CAD build for the part. Positions are in the model's coordinates, mm. A direction names the side the tool comes from. Give positions to 0.01 mm unless a question says otherwise; leave off trailing zeros. Write each loop counter-clockwise with the first axis right and the second up, starting at its lowest first coordinate (ties: lowest second). Pieces come first, ordered by that corner, then holes. Notation, with made-up numbers: (-33.5, 12.5) - (-8.5, 12.5) arc R13 cw to (-8.5, 32.5) - close; hole circle Ø7 at (44, 25.5). An arc over 180 degrees is marked (long way). Answer as a JSON object with one key per item and string values.
from build123d import *

# Parameters (mm, degrees)
SKETCH1_W           = 120
SKETCH1_H           = 40
BOSS_EXTRUDE1_DEPTH = 40
SHELL1_T            = -2
SKETCH2_R           = 18
CUT_EXTRUDE1_DEPTH  = 3
CUT_EXTRUDE2_REACH  = 42
SKETCH3_W           = 30
SKETCH3_H           = 36


with BuildPart() as part:
    # Sketch1 → Boss-Extrude1 (new body)
    with BuildSketch(Plane(origin=(0, 0, 0), x_dir=(1, 0, 0), z_dir=(0, 1, 0))):
        with Locations((-60, 20)):
            Rectangle(SKETCH1_W, SKETCH1_H)
    extrude(amount=BOSS_EXTRUDE1_DEPTH)

    # Shell1
    shell1_openings = [part.faces().sort_by_distance(p)[0] for p in [
        (-120, 20, -20),
    ]]
    offset(amount=SHELL1_T, openings=shell1_openings, kind=Kind.INTERSECTION)

    # Sketch2 → Cut-Extrude1 (cut, through all)
    with BuildSketch(Plane(origin=(0, 2, 0), x_dir=(1, 0, 0), z_dir=(0, 1, 0))):
        with Locations((-20, 20)):
            Circle(SKETCH2_R)
    extrude(amount=-CUT_EXTRUDE1_DEPTH, mode=Mode.SUBTRACT)

    # Sketch3 → Cut-Extrude2 (cut, up to next)
    with BuildSketch(Plane(origin=(0, 40, 0), x_dir=(1, 0, 0), z_dir=(0, 1, 0)), mode=Mode.PRIVATE) as cut_extrude2_sk1:
        with Locations((-101, 20)):
            Rectangle(SKETCH3_W, SKETCH3_H)
    cut_extrude2_tool1 = extrude(cut_extrude2_sk1.sketch, amount=-CUT_EXTRUDE2_REACH, mode=Mode.PRIVATE) & part.part
    add(cut_extrude2_tool1.solids().sort_by_distance((-101, 40, -20))[0], mode=Mode.SUBTRACT)


solid = part.part
Item 1: Cut at A-A (x = -96.5). Give the cut face in (y, z).
Entries:
{"outline": "(0, -40) - (40, -40) - (40, -38) - (2, -38) - (2, -2) - (40, -2) - (40, 0) - (0, 0) - close"}
Item 2: Mould opens along Y. For faces 5 (the flat face through (-6, 2, -6)), 6 (the flat face through (-61, 20, -40)), 7 (the flat face through (-48, 40, -20)) say: +Y half, -Y half, draft (parallel to the pull), parting line (faces both ways), or undercut.
Entries:
{"face 5": "undercut", "face 6": "draft", "face 7": "+Y half"}
Item 3: Cut at C-C (y = 32.5). Give the cut face in (x, z), and give its area (3 significant figures).
Entries:
{"outline": "(-120, -40) - (0, -40) - (0, 0) - (-120, 0) - (-120, -2) - (-2, -2) - (-2, -38) - (-120, -38) - close", "area": "552 mm2"}
Item 4: Cut at D-D (x = -58). Give the cut face in (y, z), and give its area (3 significant figures).
Entries:
{"outline": "(0, -40) - (40, -40) - (40, 0) - (0, 0) - close; hole (2, -38) - (38, -38) - (38, -2) - (2, -2) - close", "area": "304 mm2"}
Item 5: Probe line 1 (Z direction, x = -20, y = 1.45); line 2 (X direction, y = 1.55, z = -20); line 3 (Y direction, x = -29.5, z = -4). List the from-to ranges inside material, lowest first. Write a range as from..to.
Entries:
{"line 1": "-40..-38, -2..0", "line 2": "-120..-38, -2..0", "line 3": "0..2, 38..40"}
Item 6: Cut at B-B (z = -5). Give the cut face in (x, y), and give its area (3 significant figures).
Entries:
{"outline": "(-120, 0) - (-29.95, 0) - (-29.95, 2) - (-120, 2) - close; (-120, 38) - (-116, 38) - (-116, 40) - (-120, 40) - close; (-86, 38) - (-2, 38) - (-2, 2) - (-10.05, 2) - (-10.05, 0) - (0, 0) - (0, 40) - (-86, 40) - close", "area": "452 mm2"}
Item 7: Flat gauge pin, fed straight in: P1, Ø2, axis at y = 16, z = -18.5, coming from the -X side. Where does the tip first touch, or does it go through?
Entries:
{"P1": "x = -2"}
Item 8: Which spindle directions (+Z, -Z, +X, -X, +Y, -Y) get a long thin tool onto all of the face, cutting with end or side? Do faces 1 (the flat face through (-118, 38, -20)), 2 (the flat face through (-61, 20, 0)), 3 (the flat face through (-116, 39, -20)), 4 (the cylindrical face through (-23.902, 1.014, -2.428)). Say none if no direction does.
Entries:
{"face 1": "-X", "face 2": "+Z, +X, -X, +Y, -Y", "face 3": "+Y", "face 4": "-Y"}
